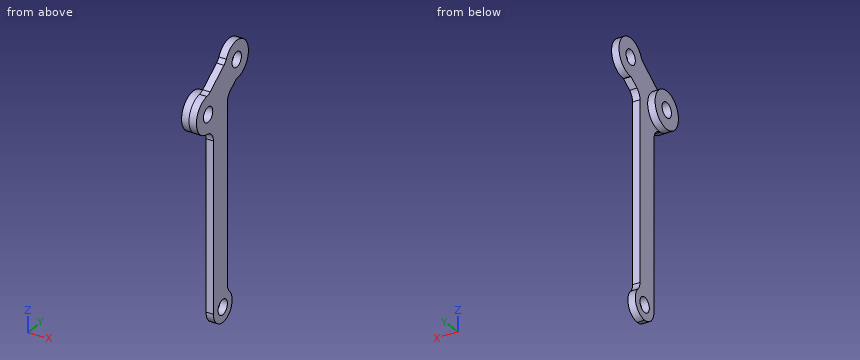
from build123d import *

# Parameters (mm, degrees)
EXTRUDE_1_DEPTH          = 2
EXTRUDE_START            = -2
SKETCH_1_4_R             = 5
EXTRUDE_2_DEPTH          = 2
CUT_EXTRUDE_1_DEPTH      = 60.733771951
CUT_EXTRUDE_1_DEPTH_BACK = 60.733771951
SKETCH_1_3_R             = 2
FILLET_1_R               = 3


with BuildPart() as part:
    # 草图1 → 凸台-拉伸1 (new body)
    with BuildSketch(Plane(origin=(0, 0, 0), x_dir=(0, 0, -1), z_dir=(1, 0, 0))):
        with BuildLine():
            Line((50.737143614, 0), (0, 0))
            Line((0, 0), (2.48051592, -3.542543867))
            ThreePointArc((2.48051592, -3.542543867), (4.165783411, -4.487079684), (5.367176995, -6))
            Line((5.367176995, -6), (54.201245229, -6))
            ThreePointArc((54.201245229, -6), (50.737143614, -4), (50.737143614, 0))
        make_face()
        with BuildLine():
            Line((2.48051592, -3.542543867), (0, 0))
            Line((0, 0), (-2.681672007, 3.829824531))
            ThreePointArc((-2.681672007, 3.829824531), (-4.811127311, -0.102785303), (-9.234888361, -0.758786959))
            Line((-9.234888361, -0.758786959), (-4.072700434, -8.131155358))
            ThreePointArc((-4.072700434, -8.131155358), (-1.94324513, -4.198545524), (2.48051592, -3.542543867))
        make_face()
        with BuildLine():
            ThreePointArc((58.201245229, -2), (55.23652141, 1.863703305), (50.737143614, 0))
            Line((50.737143614, 0), (54.201245229, 0))
            ThreePointArc((54.201245229, 0), (55.615458792, -0.585786438), (56.201245229, -2))
            ThreePointArc((56.201245229, -2), (55.615458792, -3.414213562), (54.201245229, -4))
            Line((54.201245229, -4), (54.201245229, -6))
            ThreePointArc((54.201245229, -6), (57.029672354, -4.828427125), (58.201245229, -2))
        make_face()
        with BuildLine():
            Line((54.201245229, 0), (50.737143614, 0))
            ThreePointArc((50.737143614, 0), (50.737143614, -4), (54.201245229, -6))
            Line((54.201245229, -6), (54.201245229, -4))
            ThreePointArc((54.201245229, -4), (52.201245229, -2), (54.201245229, 0))
        make_face()
        with BuildLine():
            ThreePointArc((5.367176995, -6), (4.165783411, -4.487079684), (2.48051592, -3.542543867))
            Line((2.48051592, -3.542543867), (4.201245229, -6))
            Line((4.201245229, -6), (5.367176995, -6))
        make_face()
        with BuildLine():
            Line((4.201245229, -6), (2.48051592, -3.542543867))
            ThreePointArc((2.48051592, -3.542543867), (-1.94324513, -4.198545524), (-4.072700434, -8.131155358))
            Line((-4.072700434, -8.131155358), (-2.351971125, -10.588611491))
            Line((-2.351971125, -10.588611491), (-0.713667036, -9.441458618))
            ThreePointArc((-0.713667036, -9.441458618), (-0.222515821, -6.656001657), (2.562941141, -7.147152873))
            Line((2.562941141, -7.147152873), (4.201245229, -6))
        make_face()
        with BuildLine():
            ThreePointArc((-9.234888361, -0.758786959), (-4.811127311, -0.102785303), (-2.681672007, 3.829824531))
            Line((-2.681672007, 3.829824531), (-4.402401316, 6.287280664))
            Line((-4.402401316, 6.287280664), (-6.040705405, 5.140127792))
            ThreePointArc((-6.040705405, 5.140127792), (-5.771575592, 4.594386518), (-5.679009493, 3.992974919))
            ThreePointArc((-5.679009493, 3.992974919), (-7.077597894, 2.085541017), (-9.317313582, 2.845822046))
            Line((-9.317313582, 2.845822046), (-10.95561767, 1.698669174))
            Line((-10.95561767, 1.698669174), (-9.234888361, -0.758786959))
        make_face()
        with BuildLine():
            Line((-4.402401316, 6.287280664), (-2.681672007, 3.829824531))
            ThreePointArc((-2.681672007, 3.829824531), (-2.679675166, 3.911388863), (-2.679009493, 3.992974919))
            ThreePointArc((-2.679009493, 3.992974919), (-10.613341245, 8.041394014), (-9.234888361, -0.758786959))
            Line((-9.234888361, -0.758786959), (-10.95561767, 1.698669174))
            Line((-10.95561767, 1.698669174), (-9.317313582, 2.845822046))
            ThreePointArc((-9.317313582, 2.845822046), (-8.826162366, 5.631279008), (-6.040705405, 5.140127792))
            Line((-6.040705405, 5.140127792), (-4.402401316, 6.287280664))
        make_face()
        with BuildLine():
            ThreePointArc((56.201245229, -2), (55.615458792, -0.585786438), (54.201245229, 0))
            Line((54.201245229, 0), (54.201245229, -4))
            ThreePointArc((54.201245229, -4), (55.615458792, -3.414213562), (56.201245229, -2))
        make_face()
        with BuildLine():
            Line((54.201245229, -4), (54.201245229, 0))
            ThreePointArc((54.201245229, 0), (52.201245229, -2), (54.201245229, -4))
        make_face()
        with BuildLine():
            Line((5.367176995, -6), (4.201245229, -6))
            Line((4.201245229, -6), (2.562941141, -7.147152873))
            ThreePointArc((2.562941141, -7.147152873), (2.832070954, -7.692894146), (2.924637052, -8.294305745))
            ThreePointArc((2.924637052, -8.294305745), (1.526048651, -10.201739647), (-0.713667036, -9.441458618))
            Line((-0.713667036, -9.441458618), (-2.351971125, -10.588611491))
            Line((-2.351971125, -10.588611491), (-4.072700434, -8.131155358))
            ThreePointArc((-4.072700434, -8.131155358), (0.843050996, -13.293640073), (5.924637052, -8.294305745))
            ThreePointArc((5.924637052, -8.294305745), (5.783273678, -7.113776143), (5.367176995, -6))
        make_face()
        with BuildLine():
            ThreePointArc((2.924637052, -8.294305745), (2.832070954, -7.692894146), (2.562941141, -7.147152873))
            Line((2.562941141, -7.147152873), (-0.713667036, -9.441458618))
            ThreePointArc((-0.713667036, -9.441458618), (1.526048651, -10.201739647), (2.924637052, -8.294305745))
        make_face()
        with BuildLine():
            Line((-0.713667036, -9.441458618), (2.562941141, -7.147152873))
            ThreePointArc((2.562941141, -7.147152873), (-0.222515821, -6.656001657), (-0.713667036, -9.441458618))
        make_face()
        with BuildLine():
            ThreePointArc((-5.679009493, 3.992974919), (-5.771575592, 4.594386518), (-6.040705405, 5.140127792))
            Line((-6.040705405, 5.140127792), (-9.317313582, 2.845822046))
            ThreePointArc((-9.317313582, 2.845822046), (-7.077597894, 2.085541017), (-5.679009493, 3.992974919))
        make_face()
        with BuildLine():
            Line((-9.317313582, 2.845822046), (-6.040705405, 5.140127792))
            ThreePointArc((-6.040705405, 5.140127792), (-8.826162366, 5.631279008), (-9.317313582, 2.845822046))
        make_face()
    extrude(amount=EXTRUDE_1_DEPTH)

    # 草图1<4> → 凸台-拉伸2 (add)
    with BuildSketch(Plane(origin=(0, 0, 0), x_dir=(0, 0, -1), z_dir=(1, 0, 0)).offset(EXTRUDE_START)):
        with Locations(Location((0.924637052, -8.294305745, 0), (0, 0, 178.130102354))):
            Circle(SKETCH_1_4_R)
    extrude(amount=EXTRUDE_2_DEPTH)

    # 草图1<3> → 切除-拉伸1 (cut, two sides: drawn at the far end of the back side and taken through both)
    with BuildSketch(Plane(origin=(0, 0, 0), x_dir=(0, 0, -1), z_dir=(1, 0, 0)).offset(-CUT_EXTRUDE_1_DEPTH_BACK)):
        with Locations((-7.679009493, 3.992974919)):
            Circle(SKETCH_1_3_R)
        with Locations((54.201245229, -2)):
            Circle(SKETCH_1_3_R)
        with Locations((0.924637052, -8.294305745)):
            Circle(SKETCH_1_3_R)
    extrude(amount=CUT_EXTRUDE_1_DEPTH + CUT_EXTRUDE_1_DEPTH_BACK, mode=Mode.SUBTRACT)

    # 圆角1
    # the kernel refuses this fillet: 3 mm, written as the material it adds along each edge
    with BuildSketch(Plane(origin=(0, -6, -5.367176995), x_dir=(0, 0, -1), z_dir=(1, 0, 0))) as fillet_1_piece_1:
        with BuildLine():
            CenterArc((3.526273997, -3), FILLET_1_R, 90, 84.939259464)
            ThreePointArc((0.53796877, -2.735364655), (0.463478447, -1.329430853), (0, 0))
            Line((0, 0), (3.526273997, 0))
        make_face()
    extrude(amount=2)
    with BuildSketch(Plane(origin=(0, 0, 0), x_dir=(0, 0, -1), z_dir=(1, 0, 0))) as fillet_1_piece_2:
        with BuildLine():
            CenterArc((FILLET_1_R * 0.520567050552, FILLET_1_R), FILLET_1_R, 215, 55)
            Line((-FILLET_1_R * 0.298584993737, FILLET_1_R * 0.426423563649), (0, 0))
            Line((0, 0), (FILLET_1_R * 0.520567050552, 0))
        make_face()
    extrude(amount=2)
    with BuildSketch(Plane(origin=(0, 0, -50.737143614), x_dir=(0, 0.7902368852402493, -0.6128014892326789), z_dir=(1, 0, 0))) as fillet_1_piece_3:
        with BuildLine():
            CenterArc((1.49141536, 2.972297887), FILLET_1_R, 217.792345701, 44.415308597)
            Line((-0.879295296, 1.133893419), (0, 0))
            ThreePointArc((0, 0), (0.542332858, 0.036936151), (1.084665716, 0))
        make_face()
    extrude(amount=2)
    with BuildSketch(Plane(origin=(0, -0.758786959, 9.234888361), x_dir=(0, -0.8191520442889745, -0.5735764363510707), z_dir=(1, 0, 0))) as fillet_1_piece_4:
        with BuildLine():
            CenterArc((0.872983346, -3), FILLET_1_R, 90, 28.955024372)
            ThreePointArc((-0.579385409, -0.375), (-0.283214788, -0.19750856), (0, 0))
            Line((0, 0), (0.872983346, 0))
        make_face()
    extrude(amount=2)
    with BuildSketch(Plane(origin=(0, -8.131155358, 4.072700434), x_dir=(0, -0.9993363396246481, -0.03642636827368134), z_dir=(1, 0, 0))) as fillet_1_piece_5:
        with BuildLine():
            CenterArc((0.897200113, -2.992846785), FILLET_1_R, 93.957436637, 28.955024372)
            Line((-0.732871014, -0.474341649), (0, 0))
            ThreePointArc((0, 0), (0.345076967, -0.011922025), (0.690153933, 0))
        make_face()
    extrude(amount=2)


solid = part.part
The listing builds one solid part. Answer for the finished solid, in the listing's coordinates (mm). Coordinates: 2 decimals unless noted, no trailing zeros. Write each loop counter-clockwise with the first axis right and the second up, starting at its lowest first coordinate (ties: lowest second). Pieces come first, ordered by that corner, then holes. Notation, with made-up numbers: (-26.75, 37) -> (-2.75, 37) arc R6 cw to (-2.75, 48) -> close; hole circle Ø4 at (32.5, -6.75). An arc over 180 degrees is marked (long way). One line per question, with ' | ' between items.
1. Section A-A (x = 1.15) is taken. Determine the outline of the cut face in (y, z).
Verdict:
outline: (-8.82, 4.05) arc R5 ccw to (-8.74, -5.91) arc R3 cw to (-6, -8.89) -> (-6, -54.2) arc R4 ccw (long way) to (0.86, -51.4) arc R3 cw to (0, -49.3) -> (0, -1.56) arc R3 cw to (1.28, 0.9) -> (3.83, 2.68) arc R5 ccw to (3.99, 2.68) arc R5 ccw (long way) to (-0.5, 9.87) arc R3 cw to (-1.47, 8.73) -> (-7.42, 4.57) arc R3 cw to start; hole circle Ø4 at (-8.29, -0.92); hole circle Ø4 at (-2, -54.2); hole circle Ø4 at (3.99, 7.68)
2. Given pin 1 Ø3 at (y, z) = (-2, -54.2) entering from +X; pin 2 Ø2 at (x, z) = (1, -17.5) entering from +Y; pin 3 Ø6.5 at (y, z) = (3.99, 7.68) entering from +X; pin 4 Ø1.6 at (x, z) = (1, -42.5) entering from -Y, each flat-ended and moving along its own axis, determine where each tip first touches the part or whether it passes through.
Verdict:
pin 1: passes through | pin 2: stops at y = 0 | pin 3: stops at x = 2 | pin 4: stops at y = -6
3. Straight lines are drawn through the part: line 1 (Y direction, x = 0.25, z = -21); line 2 (X direction, y = -5.5, z = -22); line 3 (Y direction, x = 1.15, z = -53). For each, find the intervals that lie inside material, in ascending order.
Verdict:
line 1: y = -6 to 0 | line 2: x = 0 to 2 | line 3: y = -6 to -3.6, -0.4 to 1.82
4. Section B-B (z = -48.5) is taken. Determine the outline of the cut face in (x, y).
Verdict:
outline: (0, -6) -> (2, -6) -> (2, 0) -> (0, 0) -> close
